Build history of the part. All positions in model axes, mm. Face numbers are marked on the shaded views. A direction names the side the tool comes from. Round coordinates to 2 decimals unless told otherwise and drop trailing zeros. Loops run counter-clockwise (first coordinate to the right, second up) from the corner with the lowest first, then second, coordinate; pieces in that order, holes last. Notation, with made-up numbers: (41.25, -13) - (87.25, -13) arc R30 ccw to (87.25, 26) - close; hole circle Ø2 at (74.5, 81). An arc over 180 degrees is marked (long way). Use a Markdown table: item, result.
from build123d import *

# Parameters (mm, degrees)
BOSS_EXTRUDE1_DEPTH      = 190
BOSS_EXTRUDE1_DEPTH_BACK = 190
SKETCH1_R                = 10.68990167
SKETCH1_R_2              = 5.55170817
SKETCH1_R_3              = 5.740939067
SKETCH1_R_4              = 6.414658556
CUT_EXTRUDE1_DEPTH       = 130
SKETCH3_R                = 6.35
BOSS_EXTRUDE2_DEPTH      = 20.842314


with BuildPart() as part:
    # Sketch1 → Boss-Extrude1 (new, two sides: drawn at the far end of the back side and taken through both)
    with BuildSketch(Plane(origin=(35.496606972, -5.136974217, 0), x_dir=(1, 0, 0), z_dir=(0, 0, 1)).offset(-BOSS_EXTRUDE1_DEPTH_BACK)):
        Polygon((298.05126311, -7.040344443), (468.668102698, -7.040344443), (468.668102698, 42.23937617), (483.730976142, 43.43752253), (505.436181993, 59.305899042), (505.436181993, 68.294900601), (519.153293081, 89.155402568), (519.153293081, 174.760868396), (511.650398428, 218.625107166), (499.221965558, 234.051088018), (499.221965558, 262.010224281), (468.239986725, 300.464582706), (385.211765775, 340.848977513), (272.476434341, 375.539814705), (268.552869962, 390.26169862), (290.33684476, 414.625354644), (269.809144882, 491.648791872), (224.483340249, 521.453400518), (173.444905467, 537.158911905), (139.442820163, 537.158911905), (39.692575389, 503.086502617), (10.46069044, 408.091209769), (22.67467758, 375.539814705), (28.02290557, 375.539814705), (66.468894181, 327.821241466), (78.40300996, 283.042400046), (93.703979809, 294.228727981), (131.920372994, 241.955284607), (123.793017705, 236.013487296), (123.793017705, 225.161132619), (105.912703634, 212.089081713), (105.912703634, 164.144657424), (139.442820163, 164.144657424), (139.442820163, 119.380028144), (217.501813233, 49.586104929), (217.501813233, 15.607484417), (284.999883711, 15.607484417), align=None)
        with Locations((129.793078962, 202.791946132)):
            Circle(SKETCH1_R, mode=Mode.SUBTRACT)
        with Locations((296.941277772, 67.915461322)):
            Circle(SKETCH1_R_2, mode=Mode.SUBTRACT)
        with Locations((487.038630051, 66.43854159)):
            Circle(SKETCH1_R_3, mode=Mode.SUBTRACT)
        with Locations((484.662417632, 257.915461322)):
            Circle(SKETCH1_R_4, mode=Mode.SUBTRACT)
    extrude(amount=BOSS_EXTRUDE1_DEPTH + BOSS_EXTRUDE1_DEPTH_BACK)

    # Sketch2 → Cut-Extrude1 (cut)
    with BuildSketch(Plane.XY.offset(190)):
        Polygon((418.856289876, -12.17731866), (418.856289876, 350.274106715), (582.658710341, 350.274106715), (582.658710341, -17.845830548), (418.856289876, -17.845830548), align=None)
    extrude(amount=-CUT_EXTRUDE1_DEPTH, mode=Mode.SUBTRACT)

    # Sketch3 → Boss-Extrude2 (add)
    with BuildSketch(Plane.XY.offset(60)):
        with Locations(Location((488.022362989, 177.803201914, 0), (0, 0, 180))):
            Circle(SKETCH3_R)
    extrude(amount=BOSS_EXTRUDE2_DEPTH)


solid = part.part
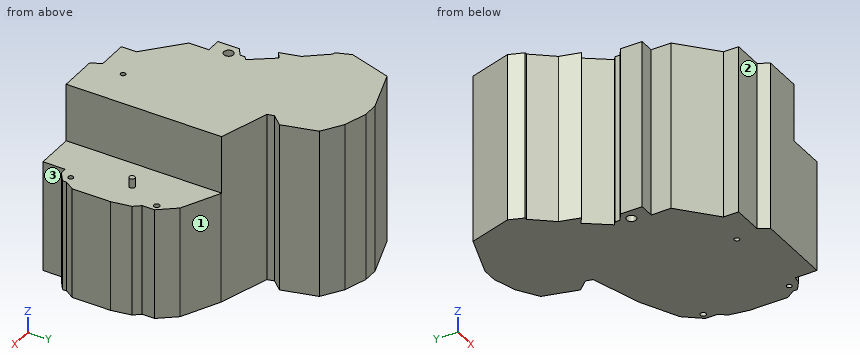
Q1. Probe line 1 (Y direction, x = 161, z = 32); line 2 (X direction, y = 120.5, z = 76); line 3 (Z direction, x = 472.5, y = 67). List the from-to ranges inside material, lowest first.
Results found:
| item | result |
|---|---|
| line 1 | y = 159.01 to 187.86, 207.45 to 232.13, 245.6 to 527.26 |
| line 2 | x = 174.94 to 418.86 |
| line 3 | z = -190 to 60 |
Q2. Cut at C-C, the plane x = 459. List the corners of the cut face in (y, z), plus the area to 3 significant figures.
Results found:
| item | result |
|---|---|
| outline | (-12.18, -190) - (317.09, -190) - (317.09, 60) - (-12.18, 60) - close |
| area | 82,300 mm2 |
Q3. Which spindle directions (+Z, -Z, +X, -X, +Y, -Y) get a long thin tool onto all of the face, cutting with end or side? Do the marked faces 1, 2 and 3. Say none if no direction does.
Results found:
| item | result |
|---|---|
| face 1 | +Z, -Z, +X, +Y |
| face 2 | +Z, -Z, -X, -Y |
| face 3 | +Z, -Z, +X, -Y |
Q4. Cut at A-A, the plane z = 165.5. Count the separate pieces of the cut face and the enclosed holes in it, plus the area to 3 significant figures.
Results found:
| item | result |
|---|---|
| separate pieces | 1 |
| enclosed holes | 2 |
| area | 129,000 mm2 |
Q5. Cut at B-B, the plane y = 148.5. List the corners of the cut face in (x, z).
Results found:
| item | result |
|---|---|
| outline | (174.94, -190) - (554.65, -190) - (554.65, 60) - (418.86, 60) - (418.86, 190) - (174.94, 190) - close |
Q6. Drop flat-ended pins along their axis: pin 1 (8.5 mm diameter, centred on y = 248.5, z = -122.5, fed in from +X); pin 2 (14.5 mm diameter, centred on y = 172, z = -7, fed in from -X); pin 3 (3 mm diameter, centred on x = 285.5, z = 127.5, fed in from -Y); pin 4 (18 mm diameter, centred on x = 332.44, y = 62.78, fed in from +Z). Give the stop position or say it passes through.
Results found:
| item | result |
|---|---|
| pin 1 | stops at x = 534.72 |
| pin 2 | stops at x = 141.41 |
| pin 3 | stops at y = 10.47 |
| pin 4 | stops at z = 190 |
